Work out the finished part from the listing and answer in its coordinate system (mm). Round coordinates to 2 decimals unless told otherwise and drop trailing zeros. Write each loop counter-clockwise with the first axis right and the second up, starting at its lowest first coordinate (ties: lowest second). Pieces come first, ordered by that corner, then holes.
1. Straight lines are drawn through the part: probe 1 along X at (y, z) = (-0.6, 146) (3 decimals); probe 2 along X at (y, z) = (-0.35, 469.9) (3 decimals); probe 3 along X at (y, z) = (-0.9, 354). For each, find the intervals that lie inside material, in ascending order.
2. Find section B-B (z = 177.5). Write down the section's boundary in (x, y) (3 decimals), and give its area (3 significant figures).
3. Find section A-A (x = -525). Write down the section's boundary in (y, z).
4. Find section C-C (y = 0.8). Count the separate pieces of the cut face and the enclosed holes in it, and give its area (3 significant figures).
```python
from build123d import *

# Parameters (mm, degrees)
F0_W     = 622.3
F0_H     = 482.6
F0_R     = 3.175
F0_R_2   = 2.579688
F1_DEPTH = 1.27
F2_W     = 34.925
F2_H     = 111.125
F2_W_2   = 6.35
F2_H_2   = 73.025
F2_H_3   = 36.5125
F2_R     = 2.579688
F3_DEPTH = 2.541


with BuildPart() as f1:
    # F0 (on Front) → F1 (new body, symmetric)
    with BuildSketch(Plane.XZ):
        with Locations((-311.15, 241.3)):
            Rectangle(F0_W, F0_H)
        with Locations((-609.6, 14.732)):
            Circle(F0_R, mode=Mode.SUBTRACT)
        with BuildLine():
            Line((-561.975, 289.306), (-561.975, 316.23))
            Line((-561.975, 316.23), (-339.725, 316.23))
            Line((-339.725, 316.23), (-339.725, 289.306))
            Line((-339.725, 289.306), (-336.55, 289.306))
            ThreePointArc((-336.55, 289.306), (-331.724, 284.48), (-336.55, 279.654))
            Line((-336.55, 279.654), (-339.725, 279.654))
            Line((-339.725, 279.654), (-339.725, 98.806))
            Line((-339.725, 98.806), (-336.55, 98.806))
            ThreePointArc((-336.55, 98.806), (-331.724, 93.98), (-336.55, 89.154))
            Line((-336.55, 89.154), (-339.725, 89.154))
            Line((-339.725, 89.154), (-339.725, 62.23))
            Line((-339.725, 62.23), (-561.975, 62.23))
            Line((-561.975, 62.23), (-561.975, 89.154))
            Line((-561.975, 89.154), (-565.15, 89.154))
            ThreePointArc((-565.15, 89.154), (-569.976, 93.98), (-565.15, 98.806))
            Line((-565.15, 98.806), (-561.975, 98.806))
            Line((-561.975, 98.806), (-561.975, 279.654))
            Line((-561.975, 279.654), (-565.15, 279.654))
            ThreePointArc((-565.15, 279.654), (-569.976, 284.48), (-565.15, 289.306))
            Line((-565.15, 289.306), (-561.975, 289.306))
        make_face(mode=Mode.SUBTRACT)
        with Locations((-311.15, 14.732)):
            Circle(F0_R, mode=Mode.SUBTRACT)
        with Locations((-12.7, 14.732)):
            Circle(F0_R, mode=Mode.SUBTRACT)
        with BuildLine():
            Line((-282.575, 62.23), (-282.575, 89.154))
            Line((-282.575, 89.154), (-285.75, 89.154))
            ThreePointArc((-285.75, 89.154), (-290.576, 93.98), (-285.75, 98.806))
            Line((-285.75, 98.806), (-282.575, 98.806))
            Line((-282.575, 98.806), (-282.575, 279.654))
            Line((-282.575, 279.654), (-285.75, 279.654))
            ThreePointArc((-285.75, 279.654), (-290.576, 284.48), (-285.75, 289.306))
            Line((-285.75, 289.306), (-282.575, 289.306))
            Line((-282.575, 289.306), (-282.575, 316.23))
            Line((-282.575, 316.23), (-60.325, 316.23))
            Line((-60.325, 316.23), (-60.325, 289.306))
            Line((-60.325, 289.306), (-57.15, 289.306))
            ThreePointArc((-57.15, 289.306), (-52.324, 284.48), (-57.15, 279.654))
            Line((-57.15, 279.654), (-60.325, 279.654))
            Line((-60.325, 279.654), (-60.325, 98.806))
            Line((-60.325, 98.806), (-57.15, 98.806))
            ThreePointArc((-57.15, 98.806), (-52.324, 93.98), (-57.15, 89.154))
            Line((-57.15, 89.154), (-60.325, 89.154))
            Line((-60.325, 89.154), (-60.325, 62.23))
            Line((-60.325, 62.23), (-282.575, 62.23))
        make_face(mode=Mode.SUBTRACT)
        with Locations((-609.6, 357.632)):
            Circle(F0_R, mode=Mode.SUBTRACT)
        with Locations((-558.8, 393.7)):
            Circle(F0_R_2, mode=Mode.SUBTRACT)
        with Locations((-558.8, 469.9)):
            Circle(F0_R_2, mode=Mode.SUBTRACT)
        with Locations((-12.7, 357.632)):
            Circle(F0_R, mode=Mode.SUBTRACT)
        with Locations((-63.5, 393.7)):
            Circle(F0_R_2, mode=Mode.SUBTRACT)
        with Locations((-63.5, 469.9)):
            Circle(F0_R_2, mode=Mode.SUBTRACT)
    extrude(amount=F1_DEPTH, both=True)

    # F2 (on face) → F3 (cut, through all)
    with BuildSketch(Plane.XZ.offset(1.27)):
        with Locations((-604.8375, 427.0375)):
            Rectangle(F2_W, F2_H)
        with Locations((-17.4625, 427.0375)):
            Rectangle(F2_W, F2_H)
        with Locations((-485.775, 352.7425)):
            Rectangle(F2_W_2, F2_H_2)
        with Locations((-415.925, 352.7425)):
            Rectangle(F2_W_2, F2_H_2)
        with Locations((-415.925, 43.97375)):
            Rectangle(F2_W_2, F2_H_3)
        with Locations((-485.775, 43.97375)):
            Rectangle(F2_W_2, F2_H_3)
        with Locations((-206.375, 352.7425)):
            Rectangle(F2_W_2, F2_H_2)
        with Locations((-136.525, 43.97375)):
            Rectangle(F2_W_2, F2_H_3)
        with Locations((-136.525, 352.7425)):
            Rectangle(F2_W_2, F2_H_2)
        with Locations((-206.375, 43.97375)):
            Rectangle(F2_W_2, F2_H_3)
        with Locations((-85.725, 441.325)):
            Circle(F2_R)
        with Locations((-536.575, 441.325)):
            Circle(F2_R)
        with Locations((-234.95, 441.325)):
            Circle(F2_R)
        with Locations((-387.35, 441.325)):
            Circle(F2_R)
    extrude(amount=-F3_DEPTH, mode=Mode.SUBTRACT)


solid = f1.part
```
Worked answers:
1. probe 1: x = -622.3 to -561.975, -339.725 to -282.575, -60.325 to 0
1. probe 2: x = -587.375 to -561.38, -556.22 to -66.08, -60.92 to -34.925
1. probe 3: x = -622.3 to -488.95, -482.6 to -419.1, -412.75 to -209.55, -203.2 to -139.7, -133.35 to 0
2. outline: (-622.3, -1.27) - (-561.975, -1.27) - (-561.975, 1.27) - (-622.3, 1.27) - close; (-339.725, -1.27) - (-282.575, -1.27) - (-282.575, 1.27) - (-339.725, 1.27) - close; (-60.325, -1.27) - (0, -1.27) - (0, 1.27) - (-60.325, 1.27) - close
2. area: 452 mm2
3. outline: (-1.27, 0) - (1.27, 0) - (1.27, 62.23) - (-1.27, 62.23) - close; (-1.27, 316.23) - (1.27, 316.23) - (1.27, 482.6) - (-1.27, 482.6) - close
4. separate pieces: 1
4. enclosed holes: 15
4. area: 176,000 mm2
